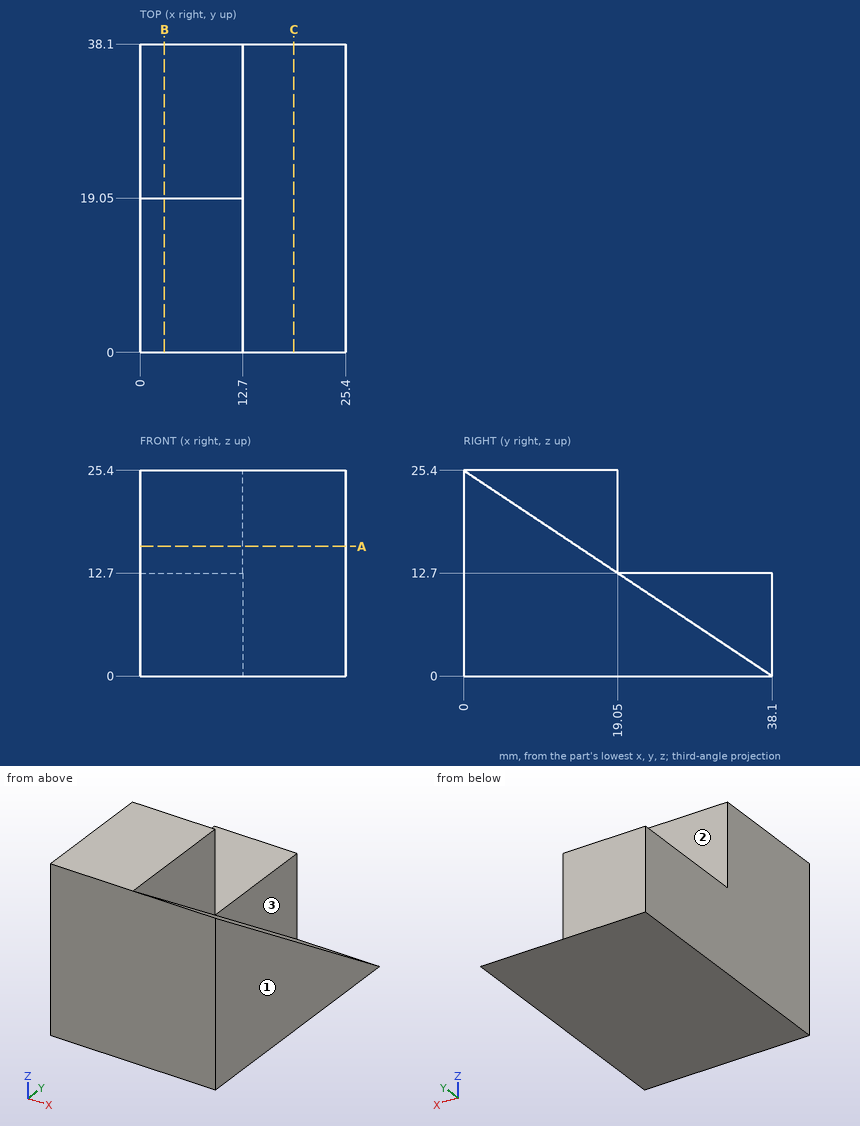
Here's the drawing with two shaded views (mm, measured from the low corner). I have some questions. A direction names the side the tool comes from. Coordinates: 2 decimals unless noted, no trailing zeros. Write each loop counter-clockwise with the first axis right and the second up, starting at its lowest first coordinate (ties: lowest second). Pieces come first, ordered by that corner, then holes. Notation, with made-up numbers: (-33, 86.5) -> (-15, 86.5) arc R32 ccw to (-15, 113.5) -> close; hole circle Ø11 at (78, -6.75). An arc over 180 degrees is marked (long way). One line per question, with ' | ' between items. Start each with the question number.
1. If we section it at B-B (x = 3): Please give me the cut outline in (y, z).
2. If we section it at A-A (z = 16): Please give me the cut outline in (x, y), and give its area (3 significant figures).
3. Will these pins go through, and if not, where does the flat tip stop? P1, Ø6, axis at x = 21.5, y = 10, coming from the +Z side; P2, Ø6.5, axis at x = 7, z = 16, coming from the +Y side; P3, Ø1, axis at x = 18.5, y = 11.5, coming from the +Z side.
4. Please list where these lines run through material, in increasing order: line 1 along Z through (x, y) = (10.5, 28); line 2 along Y through (x, z) = (18, 15.75) (3 decimals).
5. If we section it at C-C (x = 19): Please give me the cut outline in (y, z).
6. For the marked faces 1, 2 and 3, which set-ups out of +Z, -Z, +X, -X, +Y, -Y let a thin tool reach every point of the face, with its end or its side?
Return value:
1) outline: (0, 0) -> (38.1, 0) -> (38.1, 12.7) -> (19.05, 12.7) -> (19.05, 25.4) -> (0, 25.4) -> close
2) outline: (0, 0) -> (25.4, 0) -> (25.4, 14.1) -> (12.7, 14.1) -> (12.7, 19.05) -> (0, 19.05) -> close | area: 421 mm²
3) P1: stops at z = 20.73 | P2: stops at y = 19.05 | P3: stops at z = 18.07
4) line 1: z = 0 to 12.7 | line 2: y = 0 to 14.475
5) outline: (0, 0) -> (38.1, 0) -> (0, 25.4) -> close
6) face 1: +Z, -Z, +X, +Y, -Y | face 2: +Z, +X, -X, +Y | face 3: +Z, +X, +Y
